from build123d import *

# Parameters (mm, degrees)
SKETCH_1_W                  = 35
SKETCH_1_H                  = 70
EXTRUDE_1_DEPTH             = 3
CHAMFER_1_SIZE              = 4
SKETCH_2_W                  = 20.2
SKETCH_2_H                  = 40.2
CUT_EXTRUDE_1_DEPTH         = 40.246018906
SKETCH_4_R                  = 2.1
CUT_EXTRUDE_3_DEPTH         = 40.246018906
PATTERN_LINEAR_2_COUNT      = 2
PATTERN_LINEAR_2_PITCH      = 25
PATTERN_LINEAR_2_COUNT_DIR2 = 2
PATTERN_LINEAR_2_PITCH_DIR2 = 58
SKETCH_5_R                  = 2.1
CUT_EXTRUDE_4_DEPTH         = 40.246018906
PATTERN_LINEAR_3_COUNT      = 2
PATTERN_LINEAR_3_PITCH      = 10
PATTERN_LINEAR_3_COUNT_DIR2 = 2
PATTERN_LINEAR_3_PITCH_DIR2 = 50
FILLET_1_R                  = 1


with BuildPart() as part:
    # 草圖1 → 填料-伸長1 (new body)
    with BuildSketch(Plane.XY):
        Rectangle(SKETCH_1_W, SKETCH_1_H)
    extrude(amount=EXTRUDE_1_DEPTH)

    # 導角1
    chamfer_1_edges = [part.edges().sort_by_distance(p)[0] for p in [
        (17.5, -35, 1.5),
        (-17.5, -35, 1.5),
        (-17.5, 35, 1.5),
        (17.5, 35, 1.5),
    ]]
    chamfer(chamfer_1_edges, length=CHAMFER_1_SIZE)

    # 草圖2 → 除料-伸長1 (cut, through all)
    with BuildSketch(Plane(origin=(0, 0, 0), x_dir=(-1, 0, 0), z_dir=(0, 0, -1))):
        Rectangle(SKETCH_2_W, SKETCH_2_H)
    extrude(amount=-CUT_EXTRUDE_1_DEPTH, mode=Mode.SUBTRACT)

    # 草圖4 → 除料-伸長3 (cut, through all)
    with BuildSketch(Plane(origin=(0, 0, 0), x_dir=(-1, 0, 0), z_dir=(0, 0, -1))):
        with Locations((-12.5, 29)):
            Circle(SKETCH_4_R)
    cut_extrude_3 = extrude(amount=-CUT_EXTRUDE_3_DEPTH, mode=Mode.SUBTRACT)

    # 直線複製排列2: Cut-Extrude 3 2 × 2
    with Locations(*[(-i * PATTERN_LINEAR_2_PITCH, -j * PATTERN_LINEAR_2_PITCH_DIR2, 0) for i in range(PATTERN_LINEAR_2_COUNT) for j in range(PATTERN_LINEAR_2_COUNT_DIR2) if (i, j) != (0, 0)]):
        add(cut_extrude_3, mode=Mode.SUBTRACT)

    # 草圖5 → 除料-伸長4 (cut, symmetric)
    with BuildSketch(Plane.XY.offset(3)):
        with Locations((-5, -25)):
            Circle(SKETCH_5_R)
    cut_extrude_4 = extrude(amount=CUT_EXTRUDE_4_DEPTH, both=True, mode=Mode.SUBTRACT)

    # 直線複製排列3: Cut-Extrude 4 2 × 2
    with Locations(*[(i * PATTERN_LINEAR_3_PITCH, j * PATTERN_LINEAR_3_PITCH_DIR2, 0) for i in range(PATTERN_LINEAR_3_COUNT) for j in range(PATTERN_LINEAR_3_COUNT_DIR2) if (i, j) != (0, 0)]):
        add(cut_extrude_4, mode=Mode.SUBTRACT)

    # 圓角1
    fillet_1_edges = [part.edges().sort_by_distance(p)[0] for p in [
        (-10.1, 20.1, 1.5),
        (-10.1, -20.1, 1.5),
        (10.1, -20.1, 1.5),
        (10.1, 20.1, 1.5),
    ]]
    fillet(fillet_1_edges, radius=FILLET_1_R)


solid = part.part
Verification items for the finished model (mm, model axes). A direction names the side the tool comes from. Coordinates: 2 decimals unless noted, no trailing zeros. Order: outer loops, then holes, each group sorted by start corner. A loop starts at its lowest first (then second) coordinate and runs counter-clockwise, first axis right, second up. Notation, with made-up numbers: (75, 52) -> (88, 52) arc R26 cw to (88, 77) -> close; hole circle Ø9 at (15, 84). An arc over 180 degrees is marked (long way). Put each result on its own line as item: value. Start each with the question number.
1. Cross-section at C-C, the plane z = 0.55. Count the separate pieces of the cut face and the enclosed holes in it, then the cut area to 3 significant figures.
2. Cross-section at D-D, the plane x = 12.5. Record the boundary of the cut face in (y, z).
3. Cross-section at A-A, the plane x = 5. Record the boundary of the cut face in (y, z).
4. Material ranges on L1, parallel to Y at x = 12.5, z = 1.4; L2, parallel to Y at x = 5, z = 2.1; L3, parallel to Y at x = 1, z = 0.1, recorded low to high. Write a range as [from, to].
5. Mould release check, pull along Y, two halves, no side actions. Record for faces 1 (the cylindrical face through (14.6, -28.91, 1.48)), 2 (the flat face through (-17.5, 0, 1)), 3 (the cylindrical face through (6.13, -23.23, 1.52)), 4 (the flat face through (-15.5, 33, 1.5)): released by +Y, released by -Y, zero draft, split by the parting line, or undercut.
6. Access from +Z, -Z, +X, -X, +Y, -Y to the whole of each face (thin tool, end or side, straight path). Record for faces 5 (the flat face through (-10.1, 0, 1)), 6 (the flat face through (-15.5, -33, 1.5)).
7. Cross-section at B-B, the plane y = 25. Record the boundary of the cut face in (x, z).
Computed:
1. separate pieces: 1
1. enclosed holes: 9
1. area: 1,500 mm2
2. outline: (-35, 0) -> (-31.1, 0) -> (-31.1, 3) -> (-35, 3) -> close; (-26.9, 0) -> (26.9, 0) -> (26.9, 3) -> (-26.9, 3) -> close; (31.1, 0) -> (35, 0) -> (35, 3) -> (31.1, 3) -> close
3. outline: (-35, 0) -> (-27.1, 0) -> (-27.1, 3) -> (-35, 3) -> close; (-22.9, 0) -> (-20.1, 0) -> (-20.1, 3) -> (-22.9, 3) -> close; (20.1, 0) -> (22.9, 0) -> (22.9, 3) -> (20.1, 3) -> close; (27.1, 0) -> (35, 0) -> (35, 3) -> (27.1, 3) -> close
4. L1: [-35, -31.1], [-26.9, 26.9], [31.1, 35]
4. L2: [-35, -27.1], [-22.9, -20.1], [20.1, 22.9], [27.1, 35]
4. L3: [-35, -20.1], [20.1, 35]
5. face 1: undercut
5. face 2: zero draft
5. face 3: undercut
5. face 4: released by +Y
6. face 5: +Z, -Z
6. face 6: +Z, -Z, -X, -Y
7. outline: (-17.5, 0) -> (-7.1, 0) -> (-7.1, 3) -> (-17.5, 3) -> close; (-2.9, 0) -> (2.9, 0) -> (2.9, 3) -> (-2.9, 3) -> close; (7.1, 0) -> (17.5, 0) -> (17.5, 3) -> (7.1, 3) -> close
